Check sheet for the modelled part. Datum: model origin and axes. Units: mm. A direction names the side the tool comes from. Give positions to 0.01 mm unless a question says otherwise; leave off trailing zeros. Loops run counter-clockwise (first coordinate to the right, second up) from the corner with the lowest first, then second, coordinate; pieces in that order, holes last. Notation, with made-up numbers: M -29.5,19 L 3.5,19 A17 ccw 3.5,50 Z; hole C -9.75,22 d7. An arc over 180 degrees is marked long. Put each result on its own line as item: value. Start each with the question number.
Autodesk Inventor part; units mm, degrees
ref_plane "YZ Plane" through (0, 0, 0) normal (1, 0, 0) x (0, 1, 0)
ref_plane "XZ Plane" through (0, 0, 0) normal (0, 1, 0) x (-1, 0, 0)
ref_plane "XY Plane" through (0, 0, 0) normal (0, 0, 1) x (1, 0, 0)
sketch "Sketch1" plane through (0, 0, 0) normal (0, 1, 0) x (-1, 0, 0)
  line L0 (4.635, 17.27) -> (-4.635, 17.27)
  line L1 (-4.635, 17.27) -> (-4.635, -17.27)
  line L2 (-4.635, -17.27) -> (4.635, -17.27)
  line L3 (4.635, -17.27) -> (4.635, 17.27)
  point P0 (0, 0)
  dimension "d0" = 9.27
  dimension "d1" = 4.635
  dimension "d2" = 34.54
  dimension "d3" = 17.27
extrude "Extrusion1" add sketch "Sketch1" along normal blind 8.89
sketch "Sketch2" plane through (0, 0, 0) normal (0, -1, 0) x (1, 0, 0)
  line L0 (4.685, 10.79) -> (2.145, 10.79)
  line L1 (2.145, 10.79) -> (2.145, 8.25)
  line L2 (2.145, 8.25) -> (4.685, 8.25)
  line L3 (4.685, 8.25) -> (4.685, 10.79)
  line L4 (4.635, 17.27) -> (4.635, -17.27)
  line L5 (-4.635, 17.27) -> (4.635, 17.27)
  circle A0 centre (4.685, 9.52) radius 0.9772
  point P0 (0, 0)
  dimension "d6" = 2.54
  dimension "d7" = 2.54
  dimension "d8" = 0.05
  dimension "d9" = 6.48
extrude "Extrusion2" cut sketch "Sketch2" against normal blind 1.778 contours A0 L3 | L3 A0 L4 | L4 A0
pattern_linear "Rectangular Pattern1" count 6 spacing 3.81 along (0, 0, -1) of "Extrusion2"
mirror "Mirror1" about plane through (0, 0, 0) normal (1, 0, 0) of "Extrusion2", "Rectangular Pattern1"
sketch "Sketch3" plane through (0, 0, 0) normal (0, -1, 0) x (1, 0, 0)
  line L0 (1.27, -14.78) -> (-1.27, -14.78)
  line L1 (-1.27, -14.78) -> (-1.27, -17.32)
  line L2 (-1.27, -17.32) -> (1.27, -17.32)
  line L3 (1.27, -17.32) -> (1.27, -14.78)
  line L4 (4.635, -17.27) -> (-4.635, -17.27)
  circle A0 centre (0, -17.32) radius 1.0823
  point P0 (0, 0)
  dimension "d15" = 2.54
  dimension "d16" = 1.27
  dimension "d17" = 2.54
  dimension "d18" = 0.05
extrude "Extrusion3" cut sketch "Sketch3" against normal blind 1.778 contours A0 L2 L4 | L4 A0 | A0 L2
mirror "Mirror2" about plane through (0, 0, 0) normal (0, 0, 1) of "Extrusion3"
properties part number "MC_HQ1157"
Q1. Depth check by flat-ended pin: P1, Ø0.5, axis at x = -4.5, z = -2, coming from the -Y side. Enter the tip coordinate at first touch or a pass-through.
Q2. Mould release check, pull along Z, two halves, no side actions. Record for faces 1 (the face through (3.71, 0.88, -5.7)), 2 (the face through (0, 4, 17.27)), 3 (the face through (0, 1.778, 17)): pulls with the +Z half, pulls with the -Z half, needs draft (parallel to the pull), parting line crosses it, or undercut.
Q3. Section check B-B, the plane z = -1.91. Record the cut outline in (x, y) (3 decimals), then the cut area to 3 significant figures.
Q4. Access from +Z, -Z, +X, -X, +Y, -Y to the whole of each face (thin tool, end or side, straight path). Record for faces 4 (the face through (3.71, 0.88, 5.73)), 5 (the face through (4.635, 4, 0)), 6 (the face through (-0.023, 0.877, 16.238)), 7 (the face through (-3.71, 0.88, -5.74)), 8 (the face through (0, 8.89, 0)).
Found:
1. P1: stops at y = 1.78
2. face 1: undercut
2. face 2: pulls with the +Z half
2. face 3: needs draft
3. outline: M -4.635,1.778 L -3.708,1.778 L -3.708,0 L 3.708,0 L 3.708,1.778 L 4.635,1.778 L 4.635,8.89 L -4.635,8.89 Z
3. area: 79.1 mm^2
4. face 4: +X, -Y
4. face 5: +Z, -Z, +X, +Y, -Y
4. face 6: +Z, -Y
4. face 7: -X, -Y
4. face 8: +Z, -Z, +X, -X, +Y
